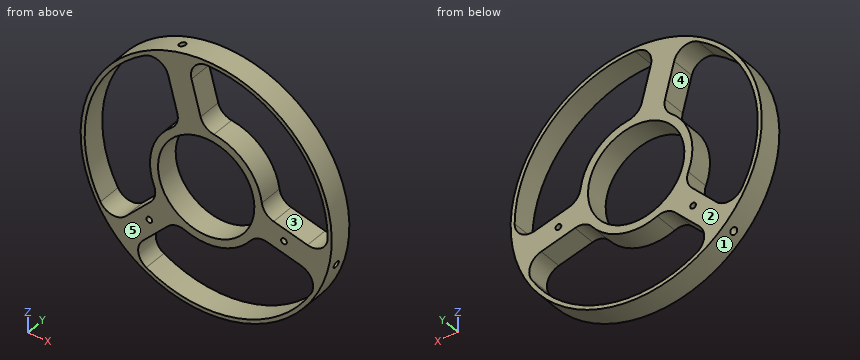
from build123d import *

# Parameters (mm, degrees)
SKETCH2_R                = 49.53
BOSS_EXTRUDE1_DEPTH      = 9.525
CUT_EXTRUDE1_REACH       = 72.691
SKETCH3_R                = 19
CIRPATTERN1_COUNT        = 3
CUT_EXTRUDE3_REACH       = 72.691
FILLET2_R                = 6.35
CIRPATTERN2_COUNT        = 3
FILLET2_OF_CIRPATTERN2_R = 6.35
F_4_40_TAPPED_HOLE1_D    = 2.2606


with BuildPart() as part:
    # Sketch2 → Boss-Extrude1 (new body)
    with BuildSketch(Plane(origin=(0, 0, 0), x_dir=(1, 0, 0), z_dir=(0, 1, 0))):
        with Locations(Location((0, 0, 0), (0, 0, 90))):
            Circle(SKETCH2_R)
    extrude(amount=BOSS_EXTRUDE1_DEPTH)

    # Sketch3 → Cut-Extrude1 (cut, up to next)
    with BuildSketch(Plane(origin=(0, 9.525, 0), x_dir=(1, 0, 0), z_dir=(0, 1, 0)), mode=Mode.PRIVATE) as cut_extrude1_sk1:
        with Locations(Location((0, 0, 0), (0, 0, 270))):
            Circle(SKETCH3_R)
    cut_extrude1_tool1 = extrude(cut_extrude1_sk1.sketch, amount=-CUT_EXTRUDE1_REACH, mode=Mode.PRIVATE) & part.part
    add(cut_extrude1_tool1.solids().sort_by_distance((0, 9.525, 0))[0], mode=Mode.SUBTRACT)

    # Sketch7 → Tap Drill for #6-32 Tap1 (revolve, cut)
    with BuildSketch(Plane(origin=(-35.022998872, 4.7625, -35.022998872), x_dir=(-0.7071067811865475, 0, 0.7071067811865476), z_dir=(0, 1, 0))):
        Polygon((0, 0), (0, 14.78269403), (1.35255, 13.97), (1.35255, 0), align=None)
    tap_drill_for_6_32_tap1 = revolve(axis=Axis((-41.488783279, 4.7625, -41.488783279), (0.7071067811865474, 0, 0.7071067811865477)), mode=Mode.SUBTRACT)

    # CirPattern1: Tap Drill for #6-32 Tap1 ×3 about axis
    cirpattern1_axis = Axis((0, -0.001, 0), (0, 1, 0))
    for i in range(1, CIRPATTERN1_COUNT):
        add(tap_drill_for_6_32_tap1.rotate(cirpattern1_axis, i * 360 / CIRPATTERN1_COUNT), mode=Mode.SUBTRACT)

    # Sketch8 → Cut-Extrude3 (cut, up to next)
    with BuildSketch(Plane(origin=(0, 9.525, 0), x_dir=(1, 0, 0), z_dir=(0, 1, 0)), mode=Mode.PRIVATE) as cut_extrude3_sk1:
        with BuildLine():
            Line((-30.365191417, 37.100383508), (-11.946600289, 18.68179238))
            ThreePointArc((-11.946600289, 18.68179238), (5.739312325, 21.419405198), (19.686955529, 10.205606645))
            Line((19.686955529, 10.205606645), (44.847218912, 16.947278899))
            ThreePointArc((44.847218912, 16.947278899), (12.40843207, 46.308898927), (-30.365191417, 37.100383508))
        make_face()
    cut_extrude3_tool1 = extrude(cut_extrude3_sk1.sketch, amount=-CUT_EXTRUDE3_REACH, mode=Mode.PRIVATE) & part.part
    cut_extrude3 = cut_extrude3_tool1.solids().sort_by_distance((8.258895, 9.525, -30.822615))[0]
    add(cut_extrude3, mode=Mode.SUBTRACT)

    # Fillet2
    fillet2_edges = [part.edges().sort_by_distance(p)[0] for p in [
        (-30.365191417, 4.7625, -37.100383508),
        (44.847218912, 4.7625, -16.947278899),
        (19.686955529, 4.7625, -10.205606645),
        (-11.946600289, 4.7625, -18.68179238),
    ]]
    fillet(fillet2_edges, radius=FILLET2_R)

    # CirPattern2: Cut-Extrude3 ×3 about axis
    cirpattern2_axis = Axis((0, 0, 0), (0, 1, 0))
    for i in range(1, CIRPATTERN2_COUNT):
        add(cut_extrude3.rotate(cirpattern2_axis, i * 360 / CIRPATTERN2_COUNT), mode=Mode.SUBTRACT)

    # Fillet2 of CirPattern2
    fillet2_of_cirpattern2_edges = [part.edges().sort_by_distance(p)[0] for p in [
        (-16.947278899, 4.7625, 44.847218912),
        (-37.100383508, 4.7625, -30.365191417),
        (-18.68179238, 4.7625, -11.946600289),
        (-10.205606645, 4.7625, 19.686955529),
        (47.312470317, 4.7625, -7.746835404),
        (-7.746835404, 4.7625, 47.312470317),
        (-1.005163149, 4.7625, 22.152206934),
        (22.152206934, 4.7625, -1.005163149),
    ]]
    fillet(fillet2_of_cirpattern2_edges, radius=FILLET2_OF_CIRPATTERN2_R)

    # #4-40 Tapped Hole1 (through all)
    with Locations(Plane(origin=(0, 9.525, 0), x_dir=(1, 0, 0), z_dir=(0, 1, 0))):
        with Locations((30.668144985, 8.217504682), (-22.450640303, 22.450640303)):
            Hole(F_4_40_TAPPED_HOLE1_D / 2)


solid = part.part
Input: part model. Units: mm. Frame: model coordinates. Face numbers are marked on the shaded views. A direction names the side the tool comes from. Give positions to 0.01 mm unless a question says otherwise; leave off trailing zeros. Write each loop counter-clockwise with the first axis right and the second up, starting at its lowest first coordinate (ties: lowest second). Pieces come first, ordered by that corner, then holes. Notation, with made-up numbers: M -39,66.25 L -8,66.25 A23 ccw -8,89.25 Z; hole C 50.25,32.25 d9. An arc over 180 degrees is marked long. Write item = value, one per line. Start each with the question number.
1) Cut plane D-D on z = 13. Return the cut outline in (x, y) (3 decimals), then the cut area to 3 significant figures.
2) First-contact query: pin 1 Ø2 at (x, y) = (-36.5, 4.5) entering from +Z; pin 2 Ø1.5 at (x, y) = (37, 8.5) entering from +Z; pin 3 Ø1 at (y, z) = (2.5, 25) entering from -X. Flat tips, straight axial feed; report the tip coordinate or a pass-through.
3) Cut plane C-C on x = -39. Return the cut outline in (y, z) (3 decimals), then the cut area to 3 significant figures.
4) Cut plane A-A on x = 7.5. Return the cut outline in (y, z) (3 decimals).
5) Material intervals for line 1 along Z through (x, y) = (-6.5, 1); line 2 along X through (y, z) = (2.5, -15.5); line 3 along Z through (x, y) = (4, 9.25), sorted ascending. Write a range as [from, to].
6) Cut plane B-B on z = -39. Return the cut outline in (x, y) (3 decimals).
7) Reachability of the marked faces 4 and 5 from +Z, -Z, +X, -X, +Y, -Y: full face, straight path, thin tool, end or side. Return the list, or none.
8) Draft query along X for the marked faces 1, 2 and 3. Return one class per face: +X half, -X half, draft (parallel to the pull), parting line (faces both ways), or undercut.
Solved:
q1.outline = M -47.794,0 L -46.146,0 L -46.146,9.525 L -47.794,9.525 Z; M -17.965,0 L -13.856,0 L -13.856,9.525 L -17.965,9.525 Z; M 13.856,0 L 17.965,0 L 17.965,9.525 L 13.856,9.525 Z; M 46.146,0 L 47.794,0 L 47.794,9.525 L 46.146,9.525 Z
q1.area = 110 mm2
q2.pin_1 = 34.54
q2.pin_2 = 33.75
q2.pin_3 = -43.05
q3.outline = M 0,-30.532 L 9.525,-30.532 L 9.525,-26.182 L 0,-26.182 Z; M 0,27.883 L 9.525,27.883 L 9.525,30.532 L 0,30.532 Z
q3.area = 66.7 mm2
q4.outline = M 0,-48.959 L 9.525,-48.959 L 9.525,-47.352 L 0,-47.352 Z; M 0,-20.868 L 9.525,-20.868 L 9.525,-17.457 L 0,-17.457 Z; M 0,17.457 L 9.525,17.457 L 9.525,20.868 L 0,20.868 Z; M 0,47.352 L 9.525,47.352 L 9.525,48.959 L 0,48.959 Z
q5.line_1 = [-49.1, -47.5], [-21.2, -17.85], [17.85, 49.1]
q5.line_2 = [-47.04, -45.37], [-22.24, -10.99], [10.99, 15.86], [38.82, 47.04]
q5.line_3 = [-49.37, -47.78], [-21.81, -18.57], [18.57, 21.81], [47.78, 49.37]
q6.outline = M -30.532,0 L -26.182,0 L -26.182,9.525 L -30.532,9.525 Z; M 27.883,0 L 30.532,0 L 30.532,9.525 L 27.883,9.525 Z
q7.face_4 = +Y, -Y
q7.face_5 = +Z, -Z, +X, -X, -Y
q8.face_1 = parting line
q8.face_2 = draft
q8.face_3 = undercut
